Part model, mm, in its own coordinate system. A direction names the side the tool comes from. Give positions to 0.01 mm unless a question says otherwise; leave off trailing zeros. Order: outer loops, then holes, each group sorted by start corner. A loop starts at its lowest first (then second) coordinate and runs counter-clockwise, first axis right, second up.
1. Drop flat-ended pins along their axis: pin 1 Ø1 at (x, y) = (12, 1.5) entering from +Z (3 decimals); pin 2 Ø1 at (y, z) = (1.5, 16.5) entering from +X. Give the stop position or say it passes through.
2. Which spindle directions (+Z, -Z, +X, -X, +Y, -Y) get a long thin tool onto all of the face, cutting with end or side? Do faces 1 (the flat face through (-11, 2, 14.865)), 2 (the flat face through (11, 2, 14.865)), 3 (the flat face through (0, 0, 8)). Say none if no direction does.
3. Probe line 1 (X direction, y = 1.45, z = 16.5); line 2 (X direction, y = 2.7, z = 13.5); line 3 (Z direction, x = 14, y = 2) (3 decimals). List the from-to ranges inside material, lowest first.
4. Slice it at C-C on z = 13. List the corners of the cut face in (x, y) (3 decimals), and give its area (3 significant figures).
5. Slice it at A-A on y = 1.1. List the corners of the cut face in (x, z) (3 decimals).
6. Slice it at B-B on x = 7.5. List the corners of the cut face in (y, z) (3 decimals), and give its area (3 significant figures).
from build123d import *

# Parameters (mm, degrees)
SKETCH1_W           = 3.175
SKETCH1_H           = 8
SKETCH1_W_2         = 30.6846
SKETCH1_H_2         = 29.73
BOSS_EXTRUDE1_DEPTH = 3.175
SKETCH2_W           = 14
SKETCH2_H           = 3.175
BOSS_EXTRUDE5_DEPTH = 3.175
SKETCH3_W           = 3.175
SKETCH3_H           = 8
SKETCH3_W_2         = 5.123924413
SKETCH3_H_2         = 0.857075887
CUT_EXTRUDE1_DEPTH  = 3.175


with BuildPart() as part:
    # Sketch1 → Boss-Extrude1 (new body)
    with BuildSketch(Plane(origin=(0, 0, 0), x_dir=(1, 0, 0), z_dir=(0, 1, 0))):
        with Locations((-16.9298, 5.865)):
            Rectangle(SKETCH1_W, SKETCH1_H)
        Rectangle(SKETCH1_W_2, SKETCH1_H_2)
        with Locations((16.9298, -5.865)):
            Rectangle(SKETCH1_W, SKETCH1_H)
        with Locations((16.9298, 5.865)):
            Rectangle(SKETCH1_W, SKETCH1_H)
        with Locations((-16.9298, -5.865)):
            Rectangle(SKETCH1_W, SKETCH1_H)
    extrude(amount=BOSS_EXTRUDE1_DEPTH)

    # Sketch2 → Boss-Extrude5 (add)
    with BuildSketch(Plane.XY.offset(14.865)):
        with Locations((0, 1.5875)):
            Rectangle(SKETCH2_W, SKETCH2_H)
    extrude(amount=BOSS_EXTRUDE5_DEPTH)

    # Sketch3 → Cut-Extrude1 (cut)
    with BuildSketch(Plane(origin=(0, 3.175, 0), x_dir=(1, 0, 0), z_dir=(0, 1, 0))):
        Polygon((-18.5173, -1.865), (-15.3423, -1.865), (-15.3423, 1.865), (-18.5173, 1.865), (-18.5173, 9.865), (-15.3423, 9.865), (-15.3423, 14.865), (-15.3423, 15.722075887), (-23.299658128, 15.722075887), (-23.299658128, -1.865), align=None)
        Polygon((-15.3423, 1.865), (-15.3423, -1.865), (-10.218375587, -1.865), (-10.218375587, 14.865), (-15.3423, 14.865), (-15.3423, 9.865), align=None)
        Polygon((-10.218375587, 14.865), (-10.218375587, -1.865), (15.3423, -1.865), (15.3423, 1.865), (18.5173, 1.865), (18.5173, 9.865), (15.3423, 9.865), (15.3423, 14.865), align=None)
        Polygon((15.3423, 1.865), (15.3423, -1.865), (18.5173, -1.865), (22.154495347, -1.865), (22.154495347, 15.722075887), (-10.218375587, 15.722075887), (-10.218375587, 14.865), (15.3423, 14.865), (15.3423, 9.865), (18.5173, 9.865), (18.5173, 1.865), align=None)
        with Locations((-16.9298, 5.865)):
            Rectangle(SKETCH3_W, SKETCH3_H)
        with Locations((-12.780337794, 15.293537944)):
            Rectangle(SKETCH3_W_2, SKETCH3_H_2)
    extrude(amount=-CUT_EXTRUDE1_DEPTH, mode=Mode.SUBTRACT)


solid = part.part
Data:
1. pin 1: stops at z = 14.865
1. pin 2: stops at x = 7
2. face 1: +Z, -X, +Y, -Y
2. face 2: +Z, +X, +Y, -Y
2. face 3: +Z, -Z, +X, -X, -Y
3. line 1: x = -7 to 7
3. line 2: x = -15.34 to 15.34
3. line 3: z = 1.865 to 14.865
4. outline: (-15.342, 0) - (15.342, 0) - (15.342, 3.175) - (-15.342, 3.175) - close
4. area: 97.4 mm2
5. outline: (-18.517, 1.865) - (18.517, 1.865) - (18.517, 9.865) - (15.342, 9.865) - (15.342, 14.865) - (7, 14.865) - (7, 18.04) - (-7, 18.04) - (-7, 14.865) - (-15.342, 14.865) - (-15.342, 9.865) - (-18.517, 9.865) - close
6. outline: (0, 1.865) - (3.175, 1.865) - (3.175, 14.865) - (0, 14.865) - close
6. area: 41.3 mm2
